Autodesk Inventor part; units mm, degrees
ref_plane "einbau_XY" through (0, 0, 0) normal (0, 0, 1) x (1, 0, 0)
ref_plane "einbau_YZ" through (0, 0, 0) normal (1, 0, 0) x (0, 1, 0)
ref_plane "einbau_ZX" through (0, 0, 0) normal (0, 1, 0) x (0, 0, 1)
sketch "Sketch_1" plane through (0, 0, 0) normal (0, 0, 1) x (1, 0, 0)
  line L0 (-34.4, 21.5) -> (-34.4, -21.5)
  arc A0 (-34.4, -21.5) -> (-28, -27.9) centre (-28, -21.5) ccw
  line L1 (-28, -27.9) -> (28, -27.9)
  arc A1 (28, -27.9) -> (34.4, -21.5) centre (28, -21.5) ccw
  line L2 (34.4, -21.5) -> (34.4, 21.5)
  arc A2 (34.4, 21.5) -> (28, 27.9) centre (28, 21.5) ccw
  line L3 (28, 27.9) -> (-28, 27.9)
  arc A3 (-28, 27.9) -> (-34.4, 21.5) centre (-28, 21.5) ccw
extrude "Extrusion1" add sketch "Sketch_1" along normal blind 0.8
sketch "Sketch_2" plane through (28, 0, 0) normal (1, 0, 0) x (0, 0, -1)
  line L0 (0, 21.5) -> (-0.8, 21.5)
  line L1 (-0.8, 21.5) -> (-0.8, 24.65)
  line L2 (-0.8, 24.65) -> (0, 23.85)
  line L3 (0, 23.85) -> (0, 21.5)
  line L4 (0, 21.5) -> (-0.8, 21.5)
revolve "Revolution1" cut sketch "Sketch_2" angle 360 about axis through (28, 21.5, 0) along (0, 0, -1)
pattern_linear "Rectangular Pattern1" count 2 spacing 56 along (-1, 0, 0) count 2 spacing 43 along (0, -1, 0) of "Revolution1"
sketch "Sketch_4" plane through (28, 0, 0) normal (1, 0, 0) x (0, 0, -1)
  line L0 (5.35, 21.5) -> (-0.65, 21.5)
  line L1 (-0.65, 21.5) -> (-0.65, 24.25)
  line L2 (-0.65, 24.25) -> (-0.25, 24.25)
  line L3 (-0.25, 24.25) -> (1, 23)
  line L4 (1, 23) -> (5.15, 23)
  line L5 (5.15, 23) -> (5.35, 22.8)
  line L6 (5.35, 22.8) -> (5.35, 21.5)
  line L7 (5.35, 21.5) -> (-0.65, 21.5)
revolve "Revolution2" add sketch "Sketch_4" angle 360 about axis through (28, 21.5, -5.35) along (0, 0, -1)
thread "Thread1"
pattern_linear "Rectangular Pattern2" count 2 spacing 56 along (-1, 0, 0) count 2 spacing 43 along (0, -1, 0) of "Revolution2"
sketch "Sketch_6" plane through (0, 0, 0.65) normal (0, 0, 1) x (1, 0, 0)
  arc A0 (27.025, 22.4093) -> (26.725, 21.8897) centre (26.875, 22.1495) ccw
  arc A1 (26.725, 21.1103) -> (26.725, 21.8897) centre (26.5, 21.5) ccw
  arc A2 (26.725, 21.1103) -> (27.025, 20.5907) centre (26.875, 20.8505) ccw
  arc A3 (27.7, 20.201) -> (27.025, 20.5907) centre (27.25, 20.201) ccw
  arc A4 (27.7, 20.201) -> (28.3, 20.201) centre (28, 20.201) ccw
  arc A5 (28.975, 20.5907) -> (28.3, 20.201) centre (28.75, 20.201) ccw
  arc A6 (28.975, 20.5907) -> (29.275, 21.1103) centre (29.125, 20.8505) ccw
  arc A7 (29.275, 21.8897) -> (29.275, 21.1103) centre (29.5, 21.5) ccw
  arc A8 (29.275, 21.8897) -> (28.975, 22.4093) centre (29.125, 22.1495) ccw
  arc A9 (28.3, 22.799) -> (28.975, 22.4093) centre (28.75, 22.799) ccw
  arc A10 (28.3, 22.799) -> (27.7, 22.799) centre (28, 22.799) ccw
  arc A11 (27.025, 22.4093) -> (27.7, 22.799) centre (27.25, 22.799) ccw
extrude "Extrusion2" cut sketch "Sketch_6" against normal blind 0.8
pattern_linear "Rectangular Pattern3" count 2 spacing 56 along (-1, 0, 0) count 2 spacing 43 along (0, -1, 0) of "Extrusion2"
ref_plane "einbau_XY" through (0, 0, 0) normal (0, 0, 1) x (1, 0, 0)
ref_plane "einbau_YZ" through (0, 0, 0) normal (1, 0, 0) x (0, 1, 0)
ref_plane "einbau_ZX" through (0, 0, 0) normal (0, 1, 0) x (0, 0, 1)
properties part number "SCHUNK-5524251 Abdeckblech-PGN-plus-P 160"
Part model, mm, in its own coordinate system. A direction names the side the tool comes from. Round coordinates to 2 decimals unless told otherwise and drop trailing zeros. Order: outer loops, then holes, each group sorted by start corner. A loop starts at its lowest first (then second) coordinate and runs counter-clockwise, first axis right, second up. Notation, with made-up numbers: M 52,-9 L 76,-9 A31 cw 76,20 Z; hole C 5,64 d2. An arc over 180 degrees is marked long. Answer in a Markdown table with one row per item. Add a question column.
Q1. 3-axis set-ups, long thin cutter, end or side, ignore diameter. For faces 1 (the face through (29.487, 21.305, -3.104)), 2 (the face through (-32.57, 25.98, 0.39)), 3 (the face through (-28, -21, -0.15)): which of +Z, -Z, +X, -X, +Y, -Y reach the whole face in a straight line?
Q2. Cut at A-A on z = -4. Give the cut face in (x, y).
Q3. Cut at C-C on x = 10.5. Give the cut face in (y, z).
Q4. Mould opens along Y. For faces 4 (the face through (32.57, -25.98, 0.39)), 5 (the face through (0, 0, 0.8)), 6 (the face through (28, 22, -0.15)) say: +Y half, -Y half, draft (parallel to the pull), parting line (faces both ways), or undercut.
Q5. Wall check: L1, parallel to Z at x = -32, y = 1.5; L2, parallel to Y at x = 27, z = -4.5; L3, parallel to Y at x = 28.5, z = -2.75. Give the ranges that are in metal, low to high. Write a range as from..to.
Q6. Cut at B-B on y = 2. Give the cut face in (x, z), and give its area (3 significant figures).
Q7. Pin check, flat tips, straight feed: pin 1 (3 mm diameter, centred on x = -29, y = -22.5, fed in from +Z); pin 2 (0.9 mm diameter, centred on x = -28.5, y = 21.5, fed in from +Z); pin 3 (4 mm diameter, centred on x = 21, y = -7.5, fed in from -Z). Stop position of each tip, or through.
Established:
| question | item | result |
|---|---|---|
| 1 | face 1 | -Z |
| 1 | face 2 | +Z, -Z, -X, +Y |
| 1 | face 3 | +Z |
| 2 | outline | C -28,-21.5 d3; C -28,21.5 d3; C 28,-21.5 d3; C 28,21.5 d3 |
| 3 | outline | M -27.9,0 L 27.9,0 L 27.9,0.8 L -27.9,0.8 Z |
| 4 | face 4 | -Y half |
| 4 | face 5 | draft |
| 4 | face 6 | undercut |
| 5 | L1 | z = 0..0.8 |
| 5 | L2 | y = -22.62..-20.38, 20.38..22.62 |
| 5 | L3 | y = -22.91..-20.09, 20.09..22.91 |
| 6 | outline | M -34.4,0 L 34.4,0 L 34.4,0.8 L -34.4,0.8 Z |
| 6 | area | 55.0 mm2 |
| 7 | pin 1 | stops at z = 0.65 |
| 7 | pin 2 | stops at z = -0.15 |
| 7 | pin 3 | stops at z = 0 |
